Here's how the part is built. I have some questions about the finished solid (model axes, mm). Face numbers are marked on the shaded views. A direction names the side the tool comes from. Give positions to 0.01 mm unless a question says otherwise; leave off trailing zeros. Write each loop counter-clockwise with the first axis right and the second up, starting at its lowest first coordinate (ties: lowest second). Pieces come first, ordered by that corner, then holes. Notation, with made-up numbers: (16.25, -33.75) -> (67.25, -33.75) arc R17 ccw to (67.25, -9.75) -> close; hole circle Ø1 at (11, 72). An arc over 180 degrees is marked (long way). Return JSON: item names as keys, results as strings.
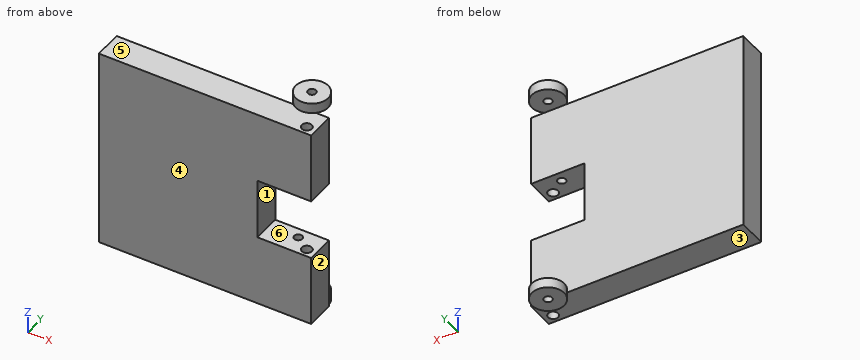
from build123d import *

# Parameters (mm, degrees)
SKETCH1_W           = 66.3702
SKETCH1_H           = 8.89
SKETCH1_R           = 1.5875
BOSS_EXTRUDE2_DEPTH = 63.5
CUT_EXTRUDE1_DEPTH  = 16.7894
SKETCH3_R           = 1.27
CUT_EXTRUDE2_DEPTH  = 12.7
CUT_EXTRUDE3_START  = -12.7
SKETCH4_R           = 1.27
CUT_EXTRUDE3_DEPTH  = 12.7
SKETCH5_R           = 5.08
SKETCH5_R_2         = 1.27
BOSS_EXTRUDE3_DEPTH = 3.175
BOSS_EXTRUDE4_START = 3.175
SKETCH6_R           = 5.08
SKETCH6_R_2         = 1.27
BOSS_EXTRUDE4_DEPTH = 3.175


with BuildPart() as part:
    # Sketch1 → Boss-Extrude2 (new body)
    with BuildSketch(Plane.XY):
        with Locations((-33.1851, 4.445)):
            Rectangle(SKETCH1_W, SKETCH1_H)
        with Locations((-2.954856457, 2.54)):
            Circle(SKETCH1_R, mode=Mode.SUBTRACT)
    extrude(amount=BOSS_EXTRUDE2_DEPTH)

    # Sketch2 → Cut-Extrude1 (cut)
    with BuildSketch(Plane(origin=(0, 0, 0), x_dir=(0, 0, -1), z_dir=(1, 0, 0))):
        Polygon((-31.75, 8.89), (-22.225, 8.89), (-22.225, 0), (-41.275, 0), (-41.275, 8.89), align=None)
    extrude(amount=-CUT_EXTRUDE1_DEPTH, mode=Mode.SUBTRACT)

    # Sketch3 → Cut-Extrude2 (cut)
    with BuildSketch(Plane(origin=(0, 0, 41.275), x_dir=(-1, 0, 0), z_dir=(0, 0, -1))):
        with Locations((7.62, 5.715)):
            Circle(SKETCH3_R)
    extrude(amount=-CUT_EXTRUDE2_DEPTH, mode=Mode.SUBTRACT)

    # Sketch4 → Cut-Extrude3 (cut)
    with BuildSketch(Plane.XY.offset(22.225).offset(CUT_EXTRUDE3_START)):
        with Locations(Location((-7.62, 5.715, 0), (0, 0, 180))):
            Circle(SKETCH4_R)
    extrude(amount=CUT_EXTRUDE3_DEPTH, mode=Mode.SUBTRACT)

    # Sketch5 → Boss-Extrude3 (add)
    with BuildSketch(Plane.XY.offset(63.5)):
        with Locations(Location((-7.62, 12.573, 0), (0, 0, 226.468847833))):
            Circle(SKETCH5_R)
        with Locations((-7.62, 12.573)):
            Circle(SKETCH5_R_2, mode=Mode.SUBTRACT)
    extrude(amount=BOSS_EXTRUDE3_DEPTH)

    # Sketch6 → Boss-Extrude4 (add)
    with BuildSketch(Plane(origin=(0, 0, 0), x_dir=(-1, 0, 0), z_dir=(0, 0, -1)).offset(BOSS_EXTRUDE4_START)):
        with Locations(Location((7.62, 12.573, 0), (0, 0, 313.531152167))):
            Circle(SKETCH6_R)
        with Locations(Location((7.62, 12.573, 0), (0, 0, 180))):
            Circle(SKETCH6_R_2, mode=Mode.SUBTRACT)
    extrude(amount=-BOSS_EXTRUDE4_DEPTH)


solid = part.part
1. If we mould it in two halves opening along Z, with no side actions, what happens to the marked faces 3, 4, 5 and 6? For each: released by +Z, released by -Z, zero draft, split by the parting line, or undercut.
Taken from the geometry:
{"face 3": "released by -Z", "face 4": "zero draft", "face 5": "released by +Z", "face 6": "undercut"}
2. Suppose I cut it at C-C, the plane z = 12. List the corners of the cut face in (x, y) for me (1 decimal), and give its area (3 significant figures).
Taken from the geometry:
{"outline": "(-66.4, 0) -> (0, 0) -> (0, 8.9) -> (-66.4, 8.9) -> close; hole circle Ø2.5 at (-7.6, 5.7); hole circle Ø3.2 at (-3, 2.5)", "area": "577 mm²"}
3. For pin 1 Ø1.5 at (x, y) = (-7.62, 12.573) entering from +Z; pin 2 Ø0.8 at (x, y) = (-7, 6) entering from -Z; pin 3 Ø6 at (x, y) = (-22.5, 4) entering from +Z; pin 4 Ø4.5 at (y, z) = (5.5, 33.5) entering from +X, each with a flat end and sliding along its axis, tell me the tip position at first contact or that it passes through.
Taken from the geometry:
{"pin 1": "passes through", "pin 2": "stops at z = 0", "pin 3": "stops at z = 63.5", "pin 4": "stops at x = -16.79"}
4. Suppose I cut it at D-D, the plane x = -62. List the corners of the cut face in (y, z) for me, and give its area (3 significant figures).
Taken from the geometry:
{"outline": "(0, 0) -> (8.89, 0) -> (8.89, 63.5) -> (0, 63.5) -> close", "area": "565 mm²"}
5. Which directions (+Z, -Z, +X, -X, +Y, -Y) give clear straight access to the entire face, cutting with the end or side of a thin tool? Please do the marked faces 1 and 2.
Taken from the geometry:
{"face 1": "+X, +Y, -Y", "face 2": "+Z, -Z, +X, +Y, -Y"}
6. If I drill on line 1 (X direction, y = 2.54, z = 13); line 2 (Y direction, x = -7.62, z = 45.5) (3 decimals); line 3 (Z direction, x = -18.5, y = 4.25), over which ranges is the centre line in solid material (lowest first)? Write a range as [from, to].
Taken from the geometry:
{"line 1": "x = [-66.37, -4.54], [-1.37, 0]", "line 2": "y = [0, 4.445], [6.985, 8.89]", "line 3": "z = [0, 63.5]"}
7. Suppose I cut it at B-B, the plane y = 2.54. List the corners of the cut face in (x, z) for me (3 decimals), and give its area (3 significant figures).
Taken from the geometry:
{"outline": "(-66.37, 0) -> (-4.542, 0) -> (-4.542, 22.225) -> (-16.789, 22.225) -> (-16.789, 41.275) -> (-4.542, 41.275) -> (-4.542, 63.5) -> (-66.37, 63.5) -> close; (-1.367, 0) -> (0, 0) -> (0, 22.225) -> (-1.367, 22.225) -> close; (-1.367, 41.275) -> (0, 41.275) -> (0, 63.5) -> (-1.367, 63.5) -> close", "area": "3,750 mm²"}
8. Suppose I cut it at A-A, the plane x = -7.62. Count the separate pieces of the cut face and the enclosed holes in it, and give its area (3 significant figures).
Taken from the geometry:
{"separate pieces": "4", "enclosed holes": "0", "area": "379 mm²"}
